Autodesk Inventor part; units mm, degrees
ref_plane "YZ Plane" through (0, 0, 0) normal (1, 0, 0) x (0, 1, 0)
ref_plane "XZ Plane" through (0, 0, 0) normal (0, 1, 0) x (-1, 0, 0)
ref_plane "XY Plane" through (0, 0, 0) normal (0, 0, 1) x (1, 0, 0)
sketch "Эскиз5" plane through (0, 0, 0) normal (0, 0, 1) x (1, 0, 0)
  line L0 (0, 0) -> (20, 0)
  line L1 (20, 0) -> (20, 25)
  line L2 (16, 29) -> (4, 29)
  line L3 (0, 25) -> (0, 0)
  line L4 (4, 29) -> (0, 25)
  line L5 (16, 29) -> (20, 25)
  point P0 (20, 29)
  point P1 (0, 29)
  dimension "d43" = 20
  dimension "d44" = 29
  dimension "d45" = 4
  dimension "d46" = 4
  dimension "d47" = 4
  dimension "d48" = 4
revolve "Вращение3" add sketch "Эскиз5" angle 360 about axis through (0, 0, 0) along (1, 0, 0)
sketch "Эскиз6" plane through (0, 0, 0) normal (-1, 0, 0) x (0, 0, 1)
  point P0 (0, 0)
  point P1 (0, 0)
hole "Отверстие3" at (0, 0, 0) direction (1, 0, 0) diameter 16 depth 9 tip angle 130 countersink diameter 18 countersink angle 90
sketch "Эскиз7" plane through (0, 0, 0) normal (-1, 0, 0) x (0, 0, 1)
  line L0 (0, 0) -> (0, 23) construction
  dimension "d57" = 23
hole "Отверстие4" at (0, 23, 0) direction (1, 0, 0) diameter 4 depth 4
sketch "Эскиз8" plane through (20, 0, 0) normal (1, 0, 0) x (0, 0, -1)
  line L0 (0, 0) -> (0, 20) construction
  dimension "d65" = 20
hole "Отверстие5" at (20, 20, 0) direction (-1, 0, 0) diameter 4 depth 4 tip angle 118
thread "Резьба3"
properties part number "711136"
Design review of the part built by this model. Coordinates are the model's own, in mm. A direction names the side the tool comes from. Give positions to 0.01 mm unless a question says otherwise; leave off trailing zeros. Order: outer loops, then holes, each group sorted by start corner. A loop starts at its lowest first (then second) coordinate and runs counter-clockwise, first axis right, second up. Notation, with made-up numbers: (83.5, 60.25) - (126.5, 60.25) arc R24 ccw to (126.5, 75.25) - close; hole circle Ø7 at (59, 53). An arc over 180 degrees is marked (long way). Use CSV: the item, a comma, the result in double quotes. Start each with the question number.
Q1. Draft analysis for pull direction Y (two halves, no side actions). For faces 4 (the face through (20, 0, 0)), 5 (the face through (2, 21, 0)), 6 (the face through (0.25, 24.084, 7.584)), state which applies: pulls with the +Y half, pulls with the -Y half, needs draft (parallel to the pull), parting line crosses it, or undercut.
Q2. Take a section at B-B (z = 0). State the section outline as (x, y) points, and give its area (3 significant figures).
Q3. For P1, Ø5, axis at x = 6.5, y = 13, coming from the +Z side; P2, Ø1, axis at x = 5, z = -1.5, coming from the +Y side; P3, Ø5, axis at x = 2, y = -19, coming from the +Z side; P4, Ø6.5, axis at y = 23, z = 0, coming from the -X side, all flat-tipped, find the tip position at first contact; note any pin that passes through.
Q4. Take a section at C-C (x = 16.75). State the section outline as (y, z) points.
Q5. Machinability: for faces 1 (the face through (18, 18, 0)), 2 (the face through (9.92, 13.38, 25.73)), 3 (the face through (4, 23, 0)), which of the approach directions +Z, -Z, +X, -X, +Y, -Y give a long, thin tool a straight path to every point of the face, cutting with its end or side? Answer none if there is none.
Q6. Take a section at D-D (x = 10.5). State the section outline as (y, z) points, and give its area (3 significant figures).
Q7. Take a section at A-A (x = 2). State the section outline as (y, z) points, and give its area (3 significant figures).
Q8. For line 1 (Y direction, x = 2.1, z = 0); line 2 (Y direction, x = 1.1, z = 0); line 3 (Z direction, x = 2.5, y = 23), list the stretches that pass through material, from the lowest coordinate up.
Calculated:
1,face 4,"needs draft"
1,face 5,"undercut"
1,face 6,"parting line crosses it"
2,outline,"(0, -25) - (4, -29) - (16, -29) - (20, -25) - (20, 18) - (16, 18) - (14.8, 20) - (16, 22) - (20, 22) - (20, 25) - (16, 29) - (4, 29) - (0, 25) - (4, 25) - (4, 21) - (0, 21) - (0, 9) - (1, 8) - (9, 8) - (12.73, 0) - (9, -8) - (1, -8) - (0, -9) - close"
2,area,"919 mm²"
3,P1,"stops at z = 27.03"
3,P2,"stops at y = 28.98"
3,P3,"stops at z = 23.12"
3,P4,"stops at x = 0"
4,outline,"circle Ø56.5 at (0, 0); hole circle Ø4 at (20, 0)"
5,face 1,"+X"
5,face 2,"+X, -X"
5,face 3,"-X"
6,outline,"circle Ø58 at (0, 0); hole circle Ø9.57 at (0, 0)"
6,area,"2,570 mm²"
7,outline,"circle Ø54 at (0, 0); hole circle Ø16 at (0, 0); hole circle Ø4 at (23, 0)"
7,area,"2,080 mm²"
8,line 1,"y = -27.1 to -8, 8 to 21, 25 to 27.1"
8,line 2,"y = -26.1 to -8, 8 to 21, 25 to 26.1"
8,line 3,"z = -15.07 to -2, 2 to 15.07"
